```python
from build123d import *

# Parameters (mm, degrees)
SKETCH1_R           = 6.75
SKETCH1_R_2         = 2.725
BOSS_EXTRUDE2_DEPTH = 10
SKETCH2_R           = 6.6
BOSS_EXTRUDE3_DEPTH = 10
CUT_EXTRUDE1_START  = -10
SKETCH3_R           = 6.6
SKETCH3_R_2         = 6.5
CUT_EXTRUDE1_DEPTH  = 10


with BuildPart() as part:
    # Sketch1 → Boss-Extrude2 (new body)
    with BuildSketch(Plane.XY):
        Circle(SKETCH1_R)
        Circle(SKETCH1_R_2, mode=Mode.SUBTRACT)
    extrude(amount=BOSS_EXTRUDE2_DEPTH)

    # Sketch2 → Boss-Extrude3 (add)
    with BuildSketch(Plane.XY.offset(10)):
        Circle(SKETCH2_R)
    extrude(amount=BOSS_EXTRUDE3_DEPTH)

    # Sketch3 → Cut-Extrude1 (cut)
    with BuildSketch(Plane.XY.offset(20).offset(CUT_EXTRUDE1_START)):
        Circle(SKETCH3_R)
        Circle(SKETCH3_R_2, mode=Mode.SUBTRACT)
    extrude(amount=CUT_EXTRUDE1_DEPTH, mode=Mode.SUBTRACT)


solid = part.part
```
Build history of the part. All positions in model axes, mm. A direction names the side the tool comes from. Give positions to 0.01 mm unless a question says otherwise; leave off trailing zeros. Order: outer loops, then holes, each group sorted by start corner. A loop starts at its lowest first (then second) coordinate and runs counter-clockwise, first axis right, second up. Notation, with made-up numbers: M 67,16 L 115,16 A26 cw 115,34 Z; hole C -29.75,2 d7. An arc over 180 degrees is marked long. Return JSON: item names as keys, results as strings.
Q1. Flat gauge pins, fed straight in: pin 1 (1.6 mm diameter, centred on x = 0.5, y = -1, fed in from -Z); pin 2 (1 mm diameter, centred on y = 3.5, z = 9.5, fed in from +X); pin 3 (4 mm diameter, centred on y = 4, z = 5.5, fed in from +X). Where does each tip first touch, or does it go through?
Answer list:
{"pin 1": "stops at z = 10", "pin 2": "stops at x = 6.05", "pin 3": "stops at x = 6.45"}
Q2. Band-saw the part on D-D (z = 12.5). Give the cut face in (x, y), then the cut area to 3 significant figures.
Answer list:
{"outline": "C 0,0 d13", "area": "133 mm^2"}
Q3. Band-saw the part on A-A (y = 0). Give the cut face in (x, z) (3 decimals).
Answer list:
{"outline": "M -6.75,0 L -2.725,0 L -2.725,10 L 2.725,10 L 2.725,0 L 6.75,0 L 6.75,10 L 6.5,10 L 6.5,20 L -6.5,20 L -6.5,10 L -6.75,10 Z"}
Q4. 3-axis set-ups, long thin cutter, end or side, ignore diameter. For faces 1 (the face through (-5.158, -3.955, 14.93)), 2 (the face through (-1.46, -6.59, 4.93)), 3 (the face through (0, 0, 10)): which of +Z, -Z, +X, -X, +Y, -Y reach the whole face in a straight line?
Answer list:
{"face 1": "+Z", "face 2": "+Z, -Z", "face 3": "-Z"}
Q5. Band-saw the part on B-B (z = 8.75). Give the cut face in (x, y) (3 decimals), then the cut area to 3 significant figures.
Answer list:
{"outline": "C 0,0 d13.5; hole C 0,0 d5.45", "area": "120 mm^2"}
Q6. Wall check: probe 1 along Y at (x, z) = (0, 3.25) (3 decimals); probe 2 along Z at (x, y) = (-1.25, 0.25); probe 3 along Y at (x, z) = (2.5, 4). Give the ranges that are in metal, low to high. Write a range as from..to.
Answer list:
{"probe 1": "y = -6.75..-2.725, 2.725..6.75", "probe 2": "z = 10..20", "probe 3": "y = -6.27..-1.08, 1.08..6.27"}
